Geometry: see drawing. Coordinates: mm, zero at the bounding-box minimum. Give positions to 0.01 mm unless a question says otherwise; leave off trailing zeros. Order: outer loops, then holes, each group sorted by start corner. A loop starts at its lowest first (then second) coordinate and runs counter-clockwise, first axis right, second up. Notation, with made-up numbers: M 70,17 L 114,17 A16 ccw 114,34 Z; hole C -31.75,-9.5 d9. An arc over 180 degrees is marked long. Return JSON: item names as keys, results as strings.
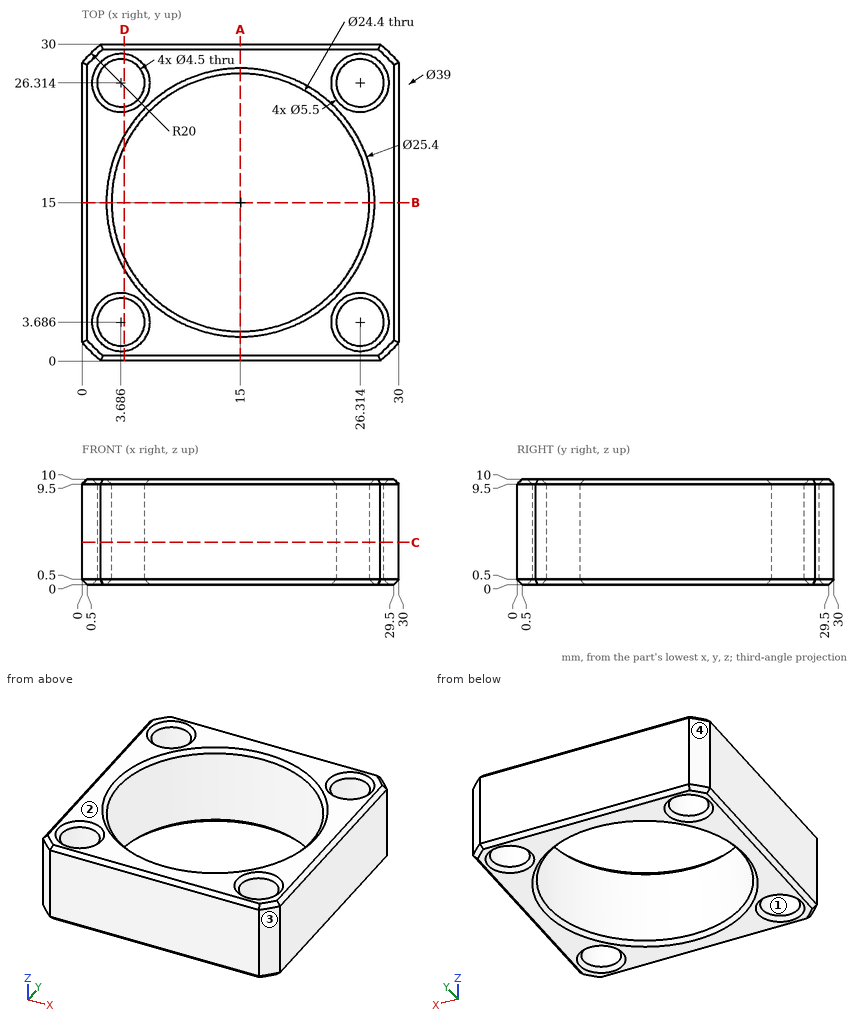
1. Section query C-C (z = 4). Return loops of the section in (x, y), then the cut area to 3 significant figures.
Evaluation:
{"outline": "M 0,1.77 A20 ccw 1.77,0 L 28.23,0 A20 ccw 30,1.77 L 30,28.23 A20 ccw 28.23,30 L 1.77,30 A20 ccw 0,28.23 Z; hole C 3.69,3.69 d4.5; hole C 3.69,26.31 d4.5; hole C 15,15 d24.4; hole C 26.31,3.69 d4.5; hole C 26.31,26.31 d4.5", "area": "363 mm^2"}
2. Section query A-A (x = 15). Return loops of the section in (y, z), then the cut area to 3 significant figures.
Evaluation:
{"outline": "M 0,0.5 L 0.5,0 L 2.3,0 L 2.8,0.5 L 2.8,9.5 L 2.3,10 L 0.5,10 L 0,9.5 Z; M 27.2,0.5 L 27.7,0 L 29.5,0 L 30,0.5 L 30,9.5 L 29.5,10 L 27.7,10 L 27.2,9.5 Z", "area": "55.0 mm^2"}
3. First-contact query: pin 1 (2 mm diameter, centred on x = 5, y = 16, fed in from +Z). Flat tip, straight axial feed; report the tip coordinate or a pass-through.
Evaluation:
{"pin 1": "passes through"}
4. Draft query along Y for the marked faces 1, 2, 3 and 4. Return one class per face: pulls with the +Y half, pulls with the -Y half, needs draft (parallel to the pull), parting line crosses it, or undercut.
Evaluation:
{"face 1": "undercut", "face 2": "needs draft", "face 3": "pulls with the -Y half", "face 4": "pulls with the +Y half"}
5. Section query D-D (x = 4). State how many separate pieces and enclosed holes the cut face has, then the cut area to 3 significant figures.
Evaluation:
{"separate pieces": "4", "enclosed holes": "0", "area": "103 mm^2"}
6. Ray query, probe 1 along X at (y, z) = (27.5, 7.5) (1 decimal); probe 2 along Y at (x, z) = (24.5, 6.25) (1 decimal); probe 3 along Y at (x, z) = (25, 9.25) (1 decimal). Return the intervals inside material, ascending.
Evaluation:
{"probe 1": "x = 0 to 1.8, 5.6 to 24.4, 28.2 to 30", "probe 2": "y = 0 to 2.4, 5 to 7.3, 22.7 to 25, 27.6 to 30", "probe 3": "y = 0 to 1.9, 5.5 to 8, 22 to 24.5, 28.1 to 30"}
